Autodesk Inventor part; units mm, degrees
ref_plane "YZ Plane" through (0, 0, 0) normal (1, 0, 0) x (0, 1, 0)
ref_plane "XZ Plane" through (0, 0, 0) normal (0, 1, 0) x (-1, 0, 0)
ref_plane "XY Plane" through (0, 0, 0) normal (0, 0, 1) x (1, 0, 0)
sketch "Sketch1" plane through (0, 0, 0) normal (0, 1, 0) x (-1, 0, 0)
  line L0 (0, 0) -> (100, 0)
  line L1 (100, 0) -> (100, -200)
  line L2 (100, -200) -> (0, -200)
  line L3 (0, -200) -> (0, 0)
  dimension "d0" = 200
  dimension "d1" = 100
extrude "Extrusion1" add sketch "Sketch1" along normal blind 6.35
sketch "Sketch2" plane through (0, 0, 0) normal (0, -1, 0) x (1, 0, 0)
  line L0 (0, 0) -> (0, -200)
  line L1 (0, -200) -> (-100, -200)
  line L2 (-100, -200) -> (-100, 0)
  line L3 (-100, 0) -> (0, 0)
  line L4 (25, 25) -> (25, -225)
  line L5 (25, -225) -> (-125, -225)
  line L6 (-125, -225) -> (-125, 25)
  line L7 (-125, 25) -> (25, 25)
  dimension "d4" = 25
extrude "Extrusion2" add sketch "Sketch2" along normal blind 10 contours L0 L1 L2 L3 | L4 L5 L6 L7
sketch "Sketch4" plane through (0, 6.35, 0) normal (0, 1, 0) x (1, 0, 0)
  line L0 (-100, 0) -> (0, 0) construction
  line L1 (-75, 0) -> (-75, 200) construction
  line L2 (0, 200) -> (-100, 200) construction
  line L3 (0, 0) -> (0, 200) construction
  line L4 (-100, 200) -> (-100, 0) construction
  line L5 (-50, 0) -> (-50, 200) construction
  line L6 (-100, 40) -> (0, 40) construction
  line L7 (-100, 120) -> (0, 120) construction
  line L8 (-100, 80) -> (0, 80) construction
  line L9 (-25, 0) -> (-25, 200) construction
  line L10 (-100, 160) -> (0, 160) construction
  circle A0 centre (-50, 120) radius 8
  circle A1 centre (-50, 80) radius 8
  circle A2 centre (-50, 40) radius 8
  circle A3 centre (-75, 160) radius 2.6
  circle A4 centre (-50, 160) radius 2.6
  circle A5 centre (-25, 160) radius 2.6
  dimension "d15" = 100
  dimension "d16" = 25
  dimension "d17" = 200
  dimension "d18" = 25
  dimension "d19" = 40
  dimension "d20" = 40
  dimension "d21" = 40
  dimension "d22" = 25
  dimension "d23" = 40
  dimension "d24" = 16
  dimension "d25" = 16
  dimension "d26" = 16
  dimension "d27" = 5.2
  dimension "d28" = 5.2
  dimension "d29" = 5.2
  dimension "d30" = 0
  dimension "d31" = 50
extrude "Extrusion3" cut sketch "Sketch4" against normal through all
sketch "Sketch5" plane through (0, -10, 0) normal (0, -1, 0) x (1, 0, 0)
  circle A0 centre (-50, -40) radius 8
  circle A1 centre (-25, -160) radius 2.6
  circle A2 centre (-50, -80) radius 8
  circle A3 centre (-75, -160) radius 2.6
  circle A4 centre (-50, -160) radius 2.6
  circle A5 centre (-50, -120) radius 8
  line L0 (0, -200) -> (-100, -200)
  line L1 (-100, -200) -> (-100, 0)
  line L2 (-100, 0) -> (0, 0)
  line L3 (0, 0) -> (0, -200)
extrude "Extrusion4" cut sketch "Sketch5" against normal blind 9.9
chamfer "Chamfer1" distance 9.9 angle 45 4 edges at (0, -0.1, -100) (-50, -0.1, 0) (-100, -0.1, -100) (-50, -0.1, -200)
sketch "Sketch9" plane through (0, -0.1, 0) normal (0, -1, 0) x (1, 0, 0)
  line L0 (-9.9, -9.9) -> (-90.1, -9.9)
  line L1 (-90.1, -9.9) -> (-90.1, -190.1)
  line L2 (-90.1, -190.1) -> (-9.9, -190.1)
  line L3 (-9.9, -190.1) -> (-9.9, -9.9)
  circle A0 centre (-50, -40) radius 8
  circle A1 centre (-25, -160) radius 2.6
  circle A2 centre (-50, -80) radius 8
  circle A3 centre (-75, -160) radius 2.6
  circle A4 centre (-50, -160) radius 2.6
  circle A5 centre (-50, -120) radius 8
  line L4 (-125, 25) -> (25, 25)
  line L5 (25, 25) -> (25, -225)
  line L6 (25, -225) -> (-125, -225)
  line L7 (-125, -225) -> (-125, 25)
  circle A6 centre (-25, -160) radius 6
  circle A7 centre (-50, -160) radius 6
  circle A8 centre (-75, -160) radius 6
  point P0 (0, 0)
  dimension "d44" = 12
  dimension "d45" = 12
  dimension "d46" = 12
extrude "Extrusion6" add sketch "Sketch9" along normal blind 5 contours A6 | A7 | A8
chamfer "Chamfer2" distance 5 angle 45 3 edges at (-31, -0.1, -160) (-56, -0.1, -160) (-81, -0.1, -160)
sketch "Sketch10" plane through (0, 6.35, 0) normal (0, 1, 0) x (1, 0, 0)
  circle A0 centre (-50, 160) radius 6
  circle A1 centre (-50, 160) radius 2.6
  circle A2 centre (-75, 160) radius 6
  circle A3 centre (-75, 160) radius 2.6
  circle A4 centre (-25, 160) radius 6
  circle A5 centre (-25, 160) radius 2.6
  point P0 (0, 0)
extrude "Extrusion7" cut sketch "Sketch10" against normal blind 8
sketch "Sketch11" plane through (0, 0, 0) normal (0, 1, 0) x (1, 0, 0)
  circle A0 centre (-25, 160) radius 6
  circle A1 centre (-50, 160) radius 6
  circle A2 centre (-75, 160) radius 6
  circle A3 centre (-50, 40) radius 8
  circle A4 centre (-50, 80) radius 8
  circle A5 centre (-50, 120) radius 8
  line L0 (-125, -25) -> (-125, 225)
  line L1 (-125, 225) -> (25, 225)
  line L2 (25, 225) -> (25, -25)
  line L3 (25, -25) -> (-125, -25)
  line L4 (0, 0) -> (0, 200)
  line L5 (0, 200) -> (-100, 200)
  line L6 (-100, 200) -> (-100, 0)
  line L7 (-100, 0) -> (0, 0)
  line L8 (-125, 200) -> (25, 200)
  line L9 (-125, 0) -> (25, 0)
extrude "Extrusion8" cut sketch "Sketch11" against normal through all contours L0 L9 L7 L2 L3 | L0 L1 L2 L8 L5
sketch "Sketch12" plane through (0, 0, 0) normal (0, 1, 0) x (1, 0, 0)
  line L0 (-125, 0) -> (-100, 0)
  line L1 (-100, 200) -> (-100, 0)
  line L2 (-100, 200) -> (-125, 200)
  line L3 (-125, 0) -> (-125, 200)
  line L4 (0, 0) -> (25, 0)
  line L5 (25, 200) -> (25, 0)
  line L6 (25, 200) -> (0, 200)
  line L7 (0, 0) -> (0, 200)
  line L8 (-112.5, 200) -> (-112.5, 0)
  line L9 (25, 200) -> (0, 200)
  line L10 (12.5, 200) -> (12.5, 0)
  line L11 (-112.5, 175) -> (12.5, 175)
  line L12 (12.5, 175) -> (12.5, 25)
  line L13 (12.5, 25) -> (-112.5, 25)
  line L14 (-112.5, 25) -> (-112.5, 175)
  point P0 (-112.5, 100)
  point P1 (12.5, 100)
  dimension "d56" = 25
  dimension "d57" = 25
hole "Hole2" at (-112.5, 0, -100) at (12.5, 0, -100) at (-112.5, 0, -175) at (12.5, 0, -175) at (12.5, 0, -25) at (-112.5, 0, -25) direction (0, -1, 0) diameter 4.69 end through all
equation "\"d16\" = 0.25 * d15"
equation "\"d18\" = d16"
equation "\"d19\" = 0.2 * d17"
equation "\"d20\" = d19"
equation "\"d21\" = d20"
equation "\"d22\" = d18"
equation "\"d23\" = d21"
equation "\"d28\" = d27"
equation "\"d29\" = d27"
equation "\"d57\" = d56"
properties part number "Faceplate"
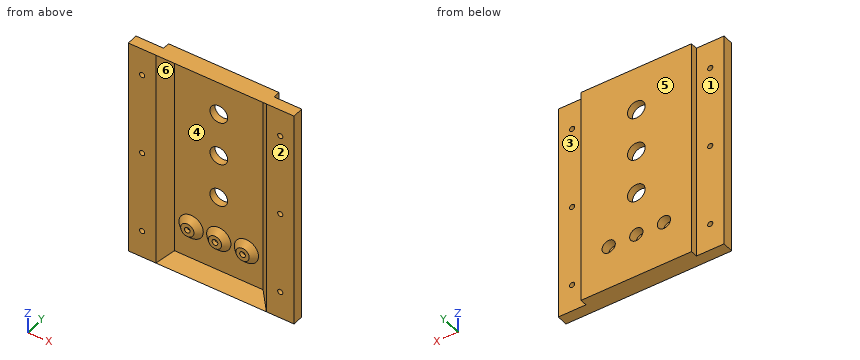
Part model, mm, in its own coordinate system. Face numbers are marked on the shaded views. A direction names the side the tool comes from. Coordinates: 2 decimals unless noted, no trailing zeros. Order: outer loops, then holes, each group sorted by start corner. A loop starts at its lowest first (then second) coordinate and runs counter-clockwise, first axis right, second up. Notation, with made-up numbers: (21, 17) -> (40, 17) arc R17 cw to (40, 44) -> close; hole circle Ø9 at (-27.5, -30). An arc over 180 degrees is marked (long way). Put each result on its own line as item: value. Start each with the question number.
(1) Band-saw the part on B-B (x = 12.5). Give the cut face in (y, z) (3 decimals), then the cut area to 3 significant figures.
(2) Pin check, flat tips, straight feed: pin 1 Ø3.5 at (x, z) = (-74, -159) entering from -Y; pin 2 Ø5 at (y, z) = (3.5, -127.5) entering from +X; pin 3 Ø8.5 at (x, z) = (-75, -160) entering from +Y. Stop position of each tip, or through.
(3) Probe line 1 along Z through (x, y) = (-50, 1.25); line 2 along Z through (x, y) = (-112.5, -5.5) (3 decimals); line 3 along X through (y, z) = (-9, -174.5). List the from-to ranges inside material, lowest first. Write a range as [from, to].
(4) Band-saw the part on A-A (x = -50). Count the separate pieces of the cut face and the enclosed holes in it, then the cut area to 3 significant figures.
(5) Which spindle directions (+Z, -Z, +X, -X, +Y, -Y) get a long thin tool onto all of the face, cutting with end or side? Do the marked faces 1, 2, 3 and 4. Say none if no direction does.
(6) Mould opens along Z. For the marked faces 5 and 6 say: pulls with the +Z half, pulls with the -Z half, needs draft (parallel to the pull), parting line crosses it, or undercut.
Determined:
1. outline: (-10, -200) -> (0, -200) -> (0, -177.345) -> (-10, -177.345) -> close; (-10, -172.655) -> (0, -172.655) -> (0, -102.345) -> (-10, -102.345) -> close; (-10, -97.655) -> (0, -97.655) -> (0, -27.345) -> (-10, -27.345) -> close; (-10, -22.655) -> (0, -22.655) -> (0, 0) -> (-10, 0) -> close
1. area: 1,860 mm²
2. pin 1: stops at y = -5.1
2. pin 2: stops at x = 0
2. pin 3: stops at y = -1.65
3. line 1: z = [-200, -166], [-154, -128], [-112, -88], [-72, -48], [-32, 0]
3. line 2: z = [-200, -177.345], [-172.655, -102.345], [-97.655, -27.345], [-22.655, 0]
3. line 3: x = [-125, -114.79], [-110.21, -99], [-1, 10.21], [14.79, 25]
4. separate pieces: 5
4. enclosed holes: 0
4. area: 1,050 mm²
5. face 1: +Z, -Z, -X, +Y
5. face 2: +Z, -Z, +X, -X, -Y
5. face 3: +Z, -Z, +X, +Y
5. face 4: -Y
6. face 5: needs draft
6. face 6: undercut
